```python
from build123d import *

# Parameters (mm, degrees)
SKETCH_1_R          = 3.5
EXTRUDE_1_DEPTH     = 1.5
SKETCH_2_R          = 1.5
EXTRUDE_2_DEPTH     = 6
FILLET_1_R          = 0.2
CUT_EXTRUDE_1_DEPTH = 1.5


with BuildPart() as part:
    # 草图1 → 凸台-拉伸1 (new body)
    with BuildSketch(Plane.XY):
        Circle(SKETCH_1_R)
    extrude(amount=EXTRUDE_1_DEPTH)

    # 草图2 → 凸台-拉伸2 (add)
    with BuildSketch(Plane.XY.offset(1.5)):
        Circle(SKETCH_2_R)
    extrude(amount=EXTRUDE_2_DEPTH)

    # 圆角1
    fillet_1_edges = [part.edges().sort_by_distance(p)[0] for p in [
        (-3.5, 0, 0),
        (-3.5, 0, 1.5),
    ]]
    fillet(fillet_1_edges, radius=FILLET_1_R)

    # 草图3 → 切除-拉伸1 (cut)
    with BuildSketch(Plane(origin=(0, 0, 0), x_dir=(-1, 0, 0), z_dir=(0, 0, -1))):
        Polygon((1.154700538, 0), (0.577350269, 1), (-0.577350269, 1), (-1.154700538, 0), (-0.577350269, -1), (0.577350269, -1), align=None)
    extrude(amount=-CUT_EXTRUDE_1_DEPTH, mode=Mode.SUBTRACT)


solid = part.part
```
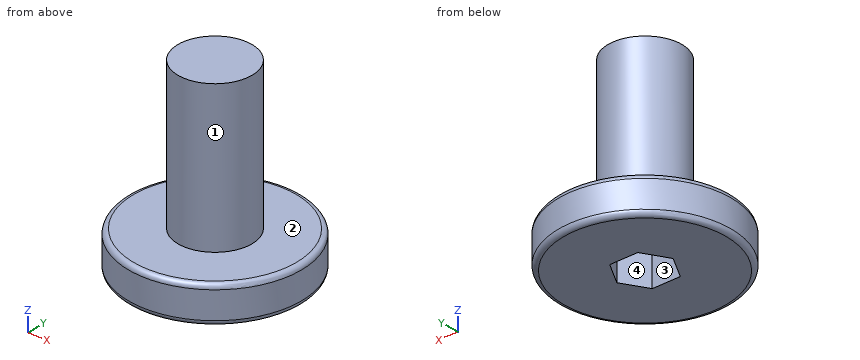
Verification items for the finished model (mm, model axes). Face numbers are marked on the shaded views. Give positions to 0.01 mm unless a question says otherwise; leave off trailing zeros. Order: outer loops, then holes, each group sorted by start corner. A loop starts at its lowest first (then second) coordinate and runs counter-clockwise, first axis right, second up. Notation, with made-up numbers: M -22,-11.75 L 33,-11.75 A9 cw 33,-6.75 Z; hole C 45,-9 d5. An arc over 180 degrees is marked long. Return JSON: item names as keys, results as strings. Group by question number.
1) Scan lines: line 1 (Z direction, x = -0.5, y = -2.5); line 2 (Y direction, x = -0.25, z = 0.5); line 3 (Y direction, x = 0, z = 5.5). Record each from-to range of solid material in increasing order.
2) Go/stop test with flat-tipped pins: pin 1 Ø1.5 at (x, z) = (2.5, 3.5) entering from +Y; pin 2 Ø0.6 at (x, z) = (-0.5, 0.5) entering from -Y. Record where each tip stops, or that it passes through.
3) Section check C-C on z = 4.75. Record the cut outline in (x, y), and give its area (3 significant figures).
4) Mould release check, pull along Y, two halves, no side actions. Record for the marked faces 1, 2, 3 and 4: pulls with the +Y half, pulls with the -Y half, needs draft (parallel to the pull), parting line crosses it, or undercut.
5) Section check B-B on x = 0. Record the cut outline in (y, z).
6) Section check A-A on z = 0.75. Record the cut outline in (x, y), and give its area (3 significant figures).
Answer block:
{
 "1": {"line 1": "z = 0 to 1.5", "line 2": "y = -3.49 to -1, 1 to 3.49", "line 3": "y = -1.5 to 1.5"},
 "2": {"pin 1": "passes through", "pin 2": "stops at y = -3.49"},
 "3": {"outline": "C 0,0 d3", "area": "7.07 mm^2"},
 "4": {"face 1": "parting line crosses it", "face 2": "needs draft", "face 3": "undercut", "face 4": "undercut"},
 "5": {"outline": "M -3.5,0.2 A0.2 ccw -3.3,0 L -1,0 L -1,1.5 L 1,1.5 L 1,0 L 3.3,0 A0.2 ccw 3.5,0.2 L 3.5,1.3 A0.2 ccw 3.3,1.5 L 1.5,1.5 L 1.5,7.5 L -1.5,7.5 L -1.5,1.5 L -3.3,1.5 A0.2 ccw -3.5,1.3 Z"},
 "6": {"outline": "C 0,0 d7; hole M -1.15,0 L -0.58,-1 L 0.58,-1 L 1.15,0 L 0.58,1 L -0.58,1 Z", "area": "35.0 mm^2"}
}
